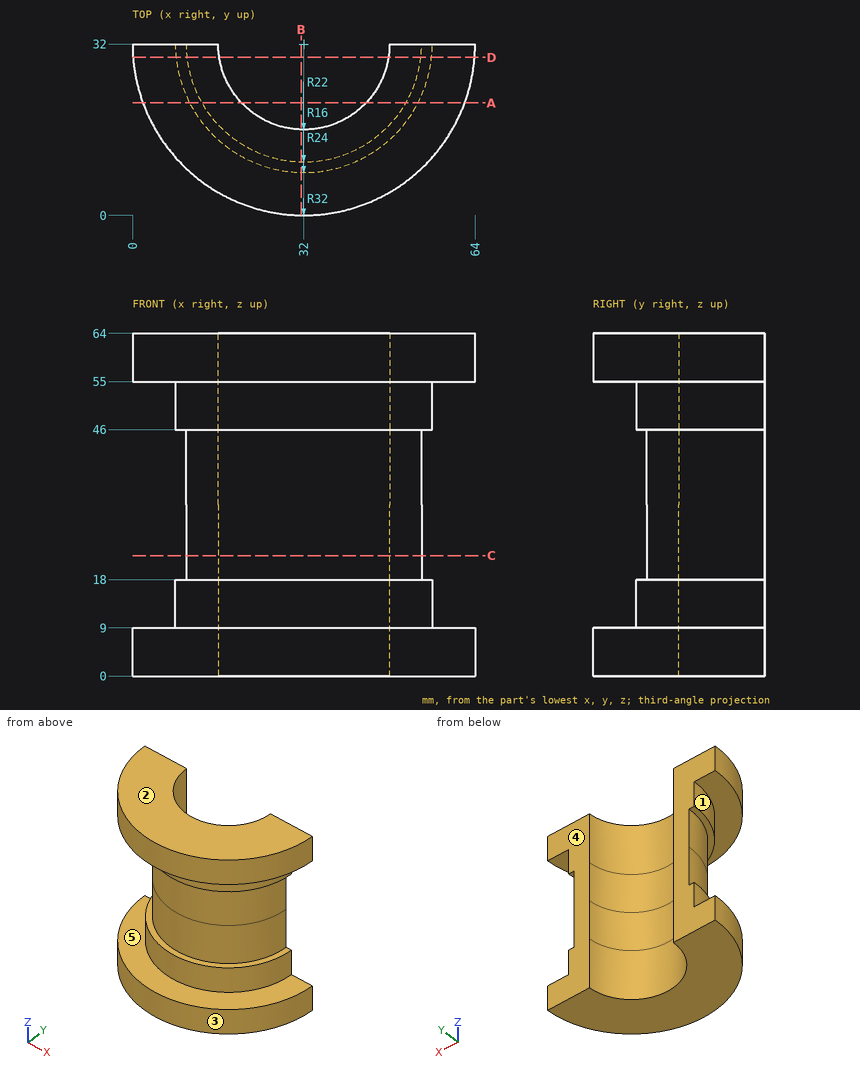
Geometry check sheet. Reference: drawing and pictorial views, mm from the part's lowest x, y, z. A direction names the side the tool comes from. Give positions to 0.01 mm unless a question says otherwise; leave off trailing zeros. Order: outer loops, then holes, each group sorted by start corner. A loop starts at its lowest first (then second) coordinate and runs counter-clockwise, first axis right, second up. Notation, with made-up numbers: (31.5, 87.5) - (38.5, 87.5) arc R34 cw to (38.5, 125.5) - close; hole circle Ø3 at (29, 10). An arc over 180 degrees is marked (long way). Answer as CSV lines item,"result". Start each with the question number.
Item 1: Section check B-B, the plane x = 31.5. Record the boundary of the cut face in (y, z), plus the area to 3 significant figures.
Item 2: Section check D-D, the plane y = 29.5. Record the boundary of the cut face in (x, z), plus the area to 3 significant figures.
Item 3: Section check C-C, the plane z = 22.5. Record the boundary of the cut face in (x, y), plus the area to 3 significant figures.
Item 4: Section check A-A, the plane y = 21. Record the boundary of the cut face in (x, z).
Item 5: Gauge pin test, flat ends, axial feed: pin 1 (6 mm diameter, centred on x = 40.5, z = 12, fed in from +Y); pin 2 (1 mm diameter, centred on y = 6, z = 53.5, fed in from -X); pin 3 (4 mm diameter, centred on x = 19, y = 8, fed in from -Z); pin 4 (8 mm diameter, centred on y = 8.5, z = 34.5, fed in from -X). Record the tip position at first contact, or that the pin passes through.
Item 6: Access from +Z, -Z, +X, -X, +Y, -Y to the whole of each face (thin tool, end or side, straight path). Record for the marked faces 4 and 5.
Item 7: Material ranges on L1, parallel to Z at x = 36, y = 7.5; L2, parallel to X at y = 27, z = 26; L3, parallel to Z at x = 29.5, y = 10, recorded low to high.
Item 8: Mould release check, pull along Z, two halves, no side actions. Record for the marked faces 1, 2 and 3: released by +Z, released by -Z, zero draft, split by the parting line, or undercut.
Filled in:
1,outline,"(0, 0) - (16.01, 0) - (16.01, 64) - (0, 64) - (0, 55) - (8.01, 55) - (8.01, 46) - (10.01, 46) - (10.01, 18) - (8.01, 18) - (8.01, 9) - (0, 9) - close"
1,area,"600 mm^2"
2,outline,"(0.1, 0) - (16.2, 0) - (16.2, 64) - (0.1, 64) - (0.1, 55) - (8.13, 55) - (8.13, 46) - (10.14, 46) - (10.14, 18) - (8.13, 18) - (8.13, 9) - (0.1, 9) - close; (47.8, 0) - (63.9, 0) - (63.9, 9) - (55.87, 9) - (55.87, 18) - (53.86, 18) - (53.86, 46) - (55.87, 46) - (55.87, 55) - (63.9, 55) - (63.9, 64) - (47.8, 64) - close"
2,area,"1,210 mm^2"
3,outline,"(10, 32) arc R22 ccw to (54, 32) - (48, 32) arc R16 cw to (16, 32) - close"
3,area,"358 mm^2"
4,outline,"(1.95, 0) - (20.38, 0) - (20.38, 64) - (1.95, 64) - (1.95, 55) - (10.67, 55) - (10.67, 46) - (12.95, 46) - (12.95, 18) - (10.67, 18) - (10.67, 9) - (1.95, 9) - close; (43.62, 0) - (62.05, 0) - (62.05, 9) - (53.33, 9) - (53.33, 18) - (51.05, 18) - (51.05, 46) - (53.33, 46) - (53.33, 55) - (62.05, 55) - (62.05, 64) - (43.62, 64) - close"
5,pin 1,"y = 20.88"
5,pin 2,"through"
5,pin 3,"z = 0"
5,pin 4,"x = 21.81"
6,face 4,"+Z, -Z, +X, -X, +Y"
6,face 5,"-Y"
7,L1,"0 to 9, 55 to 64"
7,L2,"10.58 to 16.8, 47.2 to 53.42"
7,L3,"0 to 18, 46 to 64"
8,face 1,"undercut"
8,face 2,"released by +Z"
8,face 3,"zero draft"
